from build123d import *

# Parameters (mm, degrees)
SKETCH1_W                                           = 140
SKETCH1_H                                           = 50
SKETCH1_R                                           = 5
BOSS_EXTRUDE2_DEPTH                                 = 5
CUT_EXTRUDE1_REACH                                  = 108.596
SKETCH5_R                                           = 8
CUT_EXTRUDE2_REACH                                  = 108.596
SKETCH14_R                                          = 11
CSK_FOR_M2_COUNTERSUNK_FLAT_HEAD_SCREW1_D           = 2.4
CSK_FOR_M2_COUNTERSUNK_FLAT_HEAD_SCREW1_CSINK_D     = 4.4
CSK_FOR_M2_COUNTERSUNK_FLAT_HEAD_SCREW1_CSINK_ANGLE = 90
M5_CLEARANCE_HOLE1_D                                = 5.5
M5_CLEARANCE_HOLE1_DEPTH                            = 19.75
M5_CLEARANCE_HOLE1_TIP                              = 1.652366702
CUT_EXTRUDE3_DEPTH                                  = 107.595732004


with BuildPart() as part:
    # Sketch1 → Boss-Extrude2 (new body)
    with BuildSketch(Plane(origin=(0, 0, 0), x_dir=(1, 0, 0), z_dir=(0, 1, 0))):
        with Locations((-33.501932743, 0)):
            Rectangle(SKETCH1_W, SKETCH1_H)
        with Locations(Location((16.498067257, 0, 0), (0, 0, 270))):
            Circle(SKETCH1_R, mode=Mode.SUBTRACT)
    extrude(amount=BOSS_EXTRUDE2_DEPTH)

    # Sketch5 → Cut-Extrude1 (cut, up to next)
    with BuildSketch(Plane.XZ, mode=Mode.PRIVATE) as cut_extrude1_sk1:
        with Locations(Location((-33.501932743, 0, 0), (0, 0, 270))):
            Circle(SKETCH5_R)
    cut_extrude1_tool1 = extrude(cut_extrude1_sk1.sketch, amount=-CUT_EXTRUDE1_REACH, mode=Mode.PRIVATE) & part.part
    add(cut_extrude1_tool1.solids().sort_by_distance((-33.501933, 0, 0))[0], mode=Mode.SUBTRACT)

    # Sketch14 → Cut-Extrude2 (cut, up to next)
    with BuildSketch(Plane(origin=(0, 5, 0), x_dir=(1, 0, 0), z_dir=(0, 1, 0)), mode=Mode.PRIVATE) as cut_extrude2_sk1:
        with Locations(Location((-80.801932743, 0, 0), (0, 0, 270))):
            Circle(SKETCH14_R)
    cut_extrude2_tool1 = extrude(cut_extrude2_sk1.sketch, amount=-CUT_EXTRUDE2_REACH, mode=Mode.PRIVATE) & part.part
    add(cut_extrude2_tool1.solids().sort_by_distance((-80.801933, 5, 0))[0], mode=Mode.SUBTRACT)

    # CSK for M2 Countersunk Flat Head Screw1 (through all)
    with Locations(Plane(origin=(0, 5, 0), x_dir=(1, 0, 0), z_dir=(0, 1, 0))):
        with Locations((-89.801932743, 22.5), (-71.801932743, 22.5), (-71.801932743, -22.5), (-89.801932743, -22.5), (6.498067257, 22.5), (26.498067257, 22.5), (6.498067257, -22.5), (26.498067257, -22.5)):
            CounterSinkHole(CSK_FOR_M2_COUNTERSUNK_FLAT_HEAD_SCREW1_D / 2, CSK_FOR_M2_COUNTERSUNK_FLAT_HEAD_SCREW1_CSINK_D / 2, counter_sink_angle=CSK_FOR_M2_COUNTERSUNK_FLAT_HEAD_SCREW1_CSINK_ANGLE)

    # M5 Clearance Hole1
    with Locations(Plane(origin=(0, 0, 0), x_dir=(-1, 0, 0), z_dir=(0, -1, 0))):
        with Locations((97.801932743, 15), (97.801932743, -15), (3.501932743, -15), (3.501932743, 15)):
            Hole(M5_CLEARANCE_HOLE1_D / 2, depth=M5_CLEARANCE_HOLE1_DEPTH)
            with Locations((0, 0, -(M5_CLEARANCE_HOLE1_DEPTH + M5_CLEARANCE_HOLE1_TIP / 2))):  # 118° drill point
                Cone(0, M5_CLEARANCE_HOLE1_D / 2, M5_CLEARANCE_HOLE1_TIP, mode=Mode.SUBTRACT)

    # Sketch20 → Cut-Extrude3 (cut, through all)
    with BuildSketch(Plane(origin=(0, 0, 0), x_dir=(-1, 0, 0), z_dir=(0, -1, 0))):
        with BuildLine():
            Line((46.501932743, 13), (46.501932743, 25))
            ThreePointArc((46.501932743, 25), (53.501932743, 32), (60.501932743, 25))
            Line((60.501932743, 25), (60.501932743, 13))
            ThreePointArc((60.501932743, 13), (53.501932743, 6), (46.501932743, 13))
        make_face()
    extrude(amount=-CUT_EXTRUDE3_DEPTH, mode=Mode.SUBTRACT)


solid = part.part
Could you check a few things on this model? Use its own coordinates, in mm. A direction names the side the tool comes from. Coordinates: 2 decimals unless noted, no trailing zeros. Order: outer loops, then holes, each group sorted by start corner. A loop starts at its lowest first (then second) coordinate and runs counter-clockwise, first axis right, second up. Notation, with made-up numbers: (60, -20) -> (82, -20) arc R17 cw to (82, 7) -> close; hole circle Ø5 at (-10.75, 16). An arc over 180 degrees is marked (long way). One line per item, written item: value. Start each with the question number.
1) I'm going to push flat-ended pins straight in: pin 1 (3 mm diameter, centred on x = 6.5, z = 22.5, fed in from +Y); pin 2 (4 mm diameter, centred on x = 26.5, z = -22.5, fed in from +Y). Where does each tip first touch, or does it pass through?
2) Which directions (+Z, -Z, +X, -X, +Y, -Y) give clear straight access to the entire face, cutting with the end or side of a thin tool? Please do faces 4 (the flat face through (-46.502, 2, -19)), 5 (the cylindrical face through (26.76, 1.97, 23.67)).
3) Imagine slicing it at C-C on z = 15. List the corners of the cut face in (x, y) for me, plus the area to 3 significant figures.
4) Imagine slicing it at A-A on z = -22.5. Count the separate pieces of the cut face and the enclosed holes in it, plus the area to 3 significant figures.
5) If I drill on L1, parallel to X at y = 2.55, z = -22.5; L2, parallel to X at y = 0.9, z = 22.5; L3, parallel to X at y = 1.2, z = 15, over which ranges is the centre line in solid material (lowest first)? Write a range as [from, to].
6) Imagine slicing it at D-D on x = -31. List the corners of the cut face in (y, z) for me.
7) Imagine slicing it at B-B on z = 0. List the corners of the cut face in (x, y) for me.
8) We'd pull the mould along X, two halves only. Please class faces 1 (the flat face through (36.498, 2, 0)), 2 (the cylindrical face through (-87.495, 2.535, -8.729)), 3 (the flat face through (-34, 2, 25)): +X half, -X half, draft (parallel to the pull), parting line (faces both ways), or undercut.
Answer list:
1. pin 1: stops at y = 4.3
1. pin 2: stops at y = 4.8
2. face 4: -Z, +Y, -Y
2. face 5: +Y, -Y
3. outline: (-103.5, 0) -> (-100.55, 0) -> (-100.55, 5) -> (-103.5, 5) -> close; (-95.05, 0) -> (-6.25, 0) -> (-6.25, 5) -> (-95.05, 5) -> close; (-0.75, 0) -> (36.5, 0) -> (36.5, 5) -> (-0.75, 5) -> close
3. area: 645 mm2
4. separate pieces: 6
4. enclosed holes: 0
4. area: 578 mm2
5. L1: x = [-103.5, -91], [-88.6, -73], [-70.6, -60.5], [-46.5, 5.3], [7.7, 25.3], [27.7, 36.5]
5. L2: x = [-103.5, -91], [-88.6, -73], [-70.6, 5.3], [7.7, 25.3], [27.7, 36.5]
5. L3: x = [-103.5, -100.55], [-95.05, -6.25], [-0.75, 36.5]
6. outline: (0, -25) -> (5, -25) -> (5, -7.6) -> (0, -7.6) -> close; (0, 7.6) -> (5, 7.6) -> (5, 25) -> (0, 25) -> close
7. outline: (-103.5, 0) -> (-91.8, 0) -> (-91.8, 5) -> (-103.5, 5) -> close; (-69.8, 0) -> (-41.5, 0) -> (-41.5, 5) -> (-69.8, 5) -> close; (-25.5, 0) -> (11.5, 0) -> (11.5, 5) -> (-25.5, 5) -> close; (21.5, 0) -> (36.5, 0) -> (36.5, 5) -> (21.5, 5) -> close
8. face 1: +X half
8. face 2: undercut
8. face 3: draft
